from build123d import *

# Parameters (mm, degrees)
ESQUISSE1_R           = 27
ESQUISSE1_R_2         = 15
EXTRUSION1_DEPTH      = 160
ESQUISSE2_R           = 2
EXTRUSION2_DEPTH      = 15
ESQUISSE3_R           = 2
EXTRUSION3_DEPTH      = 15
ESQUISSE4_R           = 17
ESQUISSE4_R_2         = 15
EXTRUSION4_DEPTH      = 2.5
ESQUISSE5_R           = 17
ESQUISSE5_R_2         = 15
EXTRUSION5_DEPTH      = 2.5
ESQUISSE6_W           = 120
ESQUISSE6_H           = 4.5
ESQUISSE6_H_2         = 6
EXTRUSION6_DEPTH      = 28
EXTRUSION6_DEPTH_BACK = 28


with BuildPart() as part:
    # Esquisse1 → Extrusion1 (new body)
    with BuildSketch(Plane.XY):
        Circle(ESQUISSE1_R)
        Circle(ESQUISSE1_R_2, mode=Mode.SUBTRACT)
    extrude(amount=EXTRUSION1_DEPTH)

    # Esquisse2 → Extrusion2 (cut)
    with BuildSketch(Plane.XY.offset(160)):
        with Locations((0, 24)):
            Circle(ESQUISSE2_R)
        with Locations((24, 0)):
            Circle(ESQUISSE2_R)
        with Locations((0, -24)):
            Circle(ESQUISSE2_R)
        with Locations((-24, 0)):
            Circle(ESQUISSE2_R)
    extrude(amount=-EXTRUSION2_DEPTH, mode=Mode.SUBTRACT)

    # Esquisse3 → Extrusion3 (cut)
    with BuildSketch(Plane(origin=(0, 0, 0), x_dir=(-1, 0, 0), z_dir=(0, 0, -1))):
        with Locations((0, 24)):
            Circle(ESQUISSE3_R)
        with Locations((24, 0)):
            Circle(ESQUISSE3_R)
        with Locations((0, -24)):
            Circle(ESQUISSE3_R)
        with Locations((-24, 0)):
            Circle(ESQUISSE3_R)
    extrude(amount=-EXTRUSION3_DEPTH, mode=Mode.SUBTRACT)

    # Esquisse4 → Extrusion4 (cut)
    with BuildSketch(Plane.XY.offset(160)):
        Circle(ESQUISSE4_R)
        Circle(ESQUISSE4_R_2, mode=Mode.SUBTRACT)
    extrude(amount=-EXTRUSION4_DEPTH, mode=Mode.SUBTRACT)

    # Esquisse5 → Extrusion5 (cut)
    with BuildSketch(Plane(origin=(0, 0, 0), x_dir=(-1, 0, 0), z_dir=(0, 0, -1))):
        Circle(ESQUISSE5_R)
        Circle(ESQUISSE5_R_2, mode=Mode.SUBTRACT)
    extrude(amount=-EXTRUSION5_DEPTH, mode=Mode.SUBTRACT)

    # Esquisse6 → Extrusion6 (cut, two sides)
    with BuildSketch(Plane(origin=(0, 0, 0), x_dir=(0, 0, -1), z_dir=(1, 0, 0))) as extrusion6_sk:
        with Locations((-80, 24.75)):
            Rectangle(ESQUISSE6_W, ESQUISSE6_H)
        with Locations((-80, -24)):
            Rectangle(ESQUISSE6_W, ESQUISSE6_H_2)
    extrude(amount=EXTRUSION6_DEPTH, mode=Mode.SUBTRACT)
    extrude(extrusion6_sk.sketch, amount=-EXTRUSION6_DEPTH_BACK, mode=Mode.SUBTRACT)


solid = part.part
Could you check a few things on this model? Use its own coordinates, in mm. A direction names the side the tool comes from. Round coordinates to 2 decimals unless told otherwise and drop trailing zeros. Loops run counter-clockwise (first coordinate to the right, second up) from the corner with the lowest first, then second, coordinate; pieces in that order, holes last. Notation, with made-up numbers: (-20.5, 56) - (-12.5, 56) arc R20 cw to (-12.5, 93) - close; hole circle Ø10 at (57.5, 64.25). An arc over 180 degrees is marked (long way). Write item = value, one per line.
1) If we mould it in two halves opening along Z, with no side actions, what happens to faces 6 (the flat face through (0, -23, 20)), 7 (the flat face through (0, -24, 15)), 8 (the cylindrical face through (-14.985, 0.66, 78.915)), 9 (the flat face through (0, 22.5, 81))? For each: pulls with the +Z half, pulls with the -Z half, needs draft (parallel to the pull), parting line crosses it, or undercut.
Computed:
face_6 = undercut
face_7 = pulls with the -Z half
face_8 = needs draft
face_9 = undercut
2) Imagine slicing it at C-C (x = 24). Please give me the cut outline in (y, z), and give its area (3 significant figures).
Computed:
outline = (-12.37, 0) - (-2, 0) - (-2, 15) - (2, 15) - (2, 0) - (12.37, 0) - (12.37, 160) - (2, 160) - (2, 145) - (-2, 145) - (-2, 160) - (-12.37, 160) - close
area = 3,840 mm2
3) On a 3-axis mill with a long thin cutter (end or side, diameter ignored), from which of +Z, -Z, +X, -X, +Y, -Y can I reach the whole of each face in a straight line? I mean faces 1 (the cylindrical face through (0, -22, 7)), 2 (the flat face through (18, 0, 0)), 3 (the flat face through (0, 24, 140)), 4 (the flat face through (0, -21, 81)), 5 (the flat face through (24, 0, 145)). Say none if no direction works.
Computed:
face_1 = -Z
face_2 = -Z, +X, -X, +Y, -Y
face_3 = +X, -X, +Y
face_4 = +X, -X, -Y
face_5 = +Z
4) I'm going to push flat-ended pins straight in: P1, Ø3, axis at x = 0, y = 24, coming from the +Z side; P2, Ø5, axis at x = 9.5, z = 82, coming from the -Y side; P3, Ø10, axis at y = 6, z = 119.5, coming from the -X side. Where does each tip first touch, or does it pass through?
Computed:
P1 = 145
P2 = -21
P3 = -26.98
5) Imagine slicing it at D-D (y = -24). Please give me the cut outline in (x, z), and give its area (3 significant figures).
Computed:
outline = (-12.37, 0) - (-2, 0) - (-2, 15) - (2, 15) - (2, 0) - (12.37, 0) - (12.37, 20) - (-12.37, 20) - close; (-12.37, 140) - (12.37, 140) - (12.37, 160) - (2, 160) - (2, 145) - (-2, 145) - (-2, 160) - (-12.37, 160) - close
area = 870 mm2
6) I need wall thicknesses on line 1 along Y through (x, z) = (0, 3.5); line 2 along Z through (x, y) = (8, -22.5); line 3 along X through (y, z) = (0.5, 115.5). Which ranges of each line are inside material? Lowest first, please. Write a range as from..to.
Computed:
line_1 = -27..-26, -22..-15, 15..22, 26..27
line_2 = 0..20, 140..160
line_3 = -27..-14.99, 14.99..27
7) Imagine slicing it at B-B (z = 64.5). Please give me the cut outline in (x, y), and give its area (3 significant figures).
Computed:
outline = (-16.97, -21) - (16.97, -21) arc R27 ccw to (14.92, 22.5) - (-14.92, 22.5) arc R27 ccw to start; hole circle Ø30 at (0, 0)
area = 1,350 mm2
